CAD build for the part. Positions are in the model's coordinates, mm. A direction names the side the tool comes from. Coordinates: 2 decimals unless noted, no trailing zeros. Order: outer loops, then holes, each group sorted by start corner. A loop starts at its lowest first (then second) coordinate and runs counter-clockwise, first axis right, second up. Notation, with made-up numbers: (22, 50) - (31, 50) arc R23 ccw to (31, 83) - close; hole circle Ø4 at (9, 14). An arc over 180 degrees is marked (long way). Write each question's results on one line, items separated by ' | '. Start each with the question number.
Q1. Which spindle directions (+Z, -Z, +X, -X, +Y, -Y) get a long thin tool onto all of the face, cutting with end or side? Do faces 4 (the flat face through (-24.266, 0, 2)), 5 (the flat face through (-16.556, 1, 2)), 6 (the flat face through (-1, 13, 5)), 7 (the flat face through (-19, -13.25, 2)), 8 (the flat face through (16, -18.25, 2)). Say none if no direction does.
Q2. Wall check: probe 1 along Y at (x, z) = (-0.5, 0.6); probe 2 along Y at (x, z) = (-20, 2.95); probe 3 along X at (y, z) = (10.5, 4.75). Give the ranges that are in metal, low to high.
Q3. Band-saw the part on D-D, the plane z = 3.55. Count the separate pieces of the cut face and the enclosed holes in it, then the cut area to 3 significant figures.
Q4. Pull direction Y, two halves, no side cores. Call faces 1 (the cylindrical face through (20.16, -22.65, 2.46)), 2 (the flat face through (-24.266, -20, 2)), 3 (the cylindrical face through (5.54, -14.485, 2.535)): released by +Y, released by -Y, zero draft, split by the parting line, or undercut.
Q5. Band-saw the part on A-A, the plane y = -3.5. Write the cut outline in (x, z).
Q6. Band-saw the part on C-C, the plane x = -12. Write the cut outline in (y, z), then the cut area to 3 significant figures.
Q7. Band-saw the part on B-B, the plane y = -15.75. Write the cut outline in (x, z), then the cut area to 3 significant figures.
Q8. Pin check, flat tips, straight feed: P1, Ø1.8, axis at x = -1.77, y = 25.15, coming from the -Z side; P2, Ø1.5, axis at x = 10.5, z = 2.5, coming from the +Y side. Stop position of each tip, or through.
```python
from build123d import *

# Parameters (mm, degrees)
RESSALTO_EXTRUS_O2_DEPTH = 5
ESBO_O9_W                = 29.58
ESBO_O9_H                = 18.85
CORTE_EXTRUS_O1_DEPTH    = 5
ESBO_O10_R               = 1.5
CORTE_EXTRUS_O2_DEPTH    = 5
ESBO_O12_R               = 1.5
CORTE_EXTRUS_O3_DEPTH    = 10
ESBO_O13_R               = 1.5
CORTE_EXTRUS_O4_DEPTH    = 10
ESBO_O14_R               = 1.5
CORTE_EXTRUS_O5_DEPTH    = 76


with BuildPart() as part:
    # Esboço8 → Ressalto-extrusão2 (new body)
    with BuildSketch(Plane.XY):
        with BuildLine():
            Line((-24.266341706, -3.25), (-24.266341706, 13.25))
            ThreePointArc((-24.266341706, 13.25), (-1.766341706, 35.75), (20.733658294, 13.25))
            Line((20.733658294, 13.25), (20.733658294, -3.222268622))
            Line((20.733658294, -3.222268622), (20.733658294, -3.25))
            Line((20.733658294, -3.25), (20.733658294, -13.25))
            Line((20.733658294, -13.25), (10.733658294, -13.25))
            Line((10.733658294, -13.25), (10.733658294, -18.25))
            Line((10.733658294, -18.25), (20.733658294, -18.25))
            Line((20.733658294, -18.25), (20.733658294, -21.25))
            ThreePointArc((20.733658294, -21.25), (20.147871857, -22.664213562), (18.733658294, -23.25))
            Line((18.733658294, -23.25), (-22.266341706, -23.25))
            ThreePointArc((-22.266341706, -23.25), (-23.680555268, -22.664213562), (-24.266341706, -21.25))
            Line((-24.266341706, -21.25), (-24.266341706, -18.25))
            Line((-24.266341706, -18.25), (-14.266341706, -18.25))
            Line((-14.266341706, -18.25), (-14.266341706, -13.25))
            Line((-14.266341706, -13.25), (-24.266341706, -13.25))
            Line((-24.266341706, -13.25), (-24.266341706, -3.25))
        make_face()
    extrude(amount=RESSALTO_EXTRUS_O2_DEPTH)

    # Esboço9 → Corte-extrusão1 (cut)
    with BuildSketch(Plane(origin=(0, 0, 0), x_dir=(-1, 0, 0), z_dir=(0, 0, -1))):
        with Locations((1.766341706, 1.175)):
            Rectangle(ESBO_O9_W, ESBO_O9_H)
    extrude(amount=-CORTE_EXTRUS_O1_DEPTH, mode=Mode.SUBTRACT)

    # Esboço10 → Corte-extrusão2 (cut)
    with BuildSketch(Plane(origin=(0, 0, 0), x_dir=(-1, 0, 0), z_dir=(0, 0, -1))):
        with Locations((-17.733658294, 0)):
            Circle(ESBO_O10_R)
        with Locations((21.266341706, 0)):
            Circle(ESBO_O10_R)
    extrude(amount=-CORTE_EXTRUS_O2_DEPTH, mode=Mode.SUBTRACT)

    # Esboço12 → Corte-extrusão3 (cut)
    with BuildSketch(Plane.XY.offset(5)):
        with Locations((4.733658294, -15.75)):
            Circle(ESBO_O12_R)
        with Locations((-8.266341706, -15.75)):
            Circle(ESBO_O12_R)
    extrude(amount=-CORTE_EXTRUS_O3_DEPTH, mode=Mode.SUBTRACT)

    # Esboço13 → Corte-extrusão4 (cut)
    with BuildSketch(Plane.XY.offset(5)):
        with Locations((-1.766341706, 25.15)):
            Circle(ESBO_O13_R)
    extrude(amount=-CORTE_EXTRUS_O4_DEPTH, mode=Mode.SUBTRACT)

    # Esboço14 → Corte-extrusão5 (cut)
    with BuildSketch(Plane.XY.offset(5)):
        with Locations((14.733658294, 17.25)):
            Circle(ESBO_O14_R)
        with Locations((14.733658294, 23.25)):
            Circle(ESBO_O14_R)
        with Locations((-18.266341706, 23.25)):
            Circle(ESBO_O14_R)
        with Locations((-18.266341706, 17.25)):
            Circle(ESBO_O14_R)
    extrude(amount=-CORTE_EXTRUS_O5_DEPTH, mode=Mode.SUBTRACT)


solid = part.part
```
Results below:
1) face 4: +Z, -Z, -X, +Y, -Y | face 5: +Z, -Z | face 6: +Z, +X, -X, +Y, -Y | face 7: +Z, -Z, -X | face 8: +Z, -Z, +X
2) probe 1: y = -23.25 to -8.25, 10.6 to 24.35, 25.95 to 35.71 | probe 2: y = -23.25 to -18.25, -13.25 to -0.8, 0.8 to 26.43 | probe 3: x = -24.27 to -16.56, 13.02 to 20.73
3) separate pieces: 1 | enclosed holes: 10 | area: 1,710 mm²
4) face 1: released by -Y | face 2: zero draft | face 3: undercut
5) outline: (-24.27, 0) - (-16.56, 0) - (-16.56, 5) - (-24.27, 5) - close; (13.02, 0) - (20.73, 0) - (20.73, 5) - (13.02, 5) - close
6) outline: (-23.25, 0) - (-8.25, 0) - (-8.25, 5) - (-23.25, 5) - close; (10.6, 0) - (33.29, 0) - (33.29, 5) - (10.6, 5) - close | area: 188 mm²
7) outline: (-14.27, 0) - (-9.77, 0) - (-9.77, 5) - (-14.27, 5) - close; (-6.77, 0) - (3.23, 0) - (3.23, 5) - (-6.77, 5) - close; (6.23, 0) - (10.73, 0) - (10.73, 5) - (6.23, 5) - close | area: 95.0 mm²
8) P1: passes through | P2: stops at y = 32.58
